Job drawing, mm, ordinate dimensions from the low corner. One solid piece. A direction names the side the tool comes from. Coordinates: 2 decimals unless noted, no trailing zeros. Order: outer loops, then holes, each group sorted by start corner. A loop starts at its lowest first (then second) coordinate and runs counter-clockwise, first axis right, second up. Notation, with made-up numbers: (40.5, -40) - (81.5, -40) arc R15 ccw to (81.5, -31) - close; hole circle Ø5 at (17, 88). An arc over 180 degrees is marked (long way). Use one line per item in the form item = value.
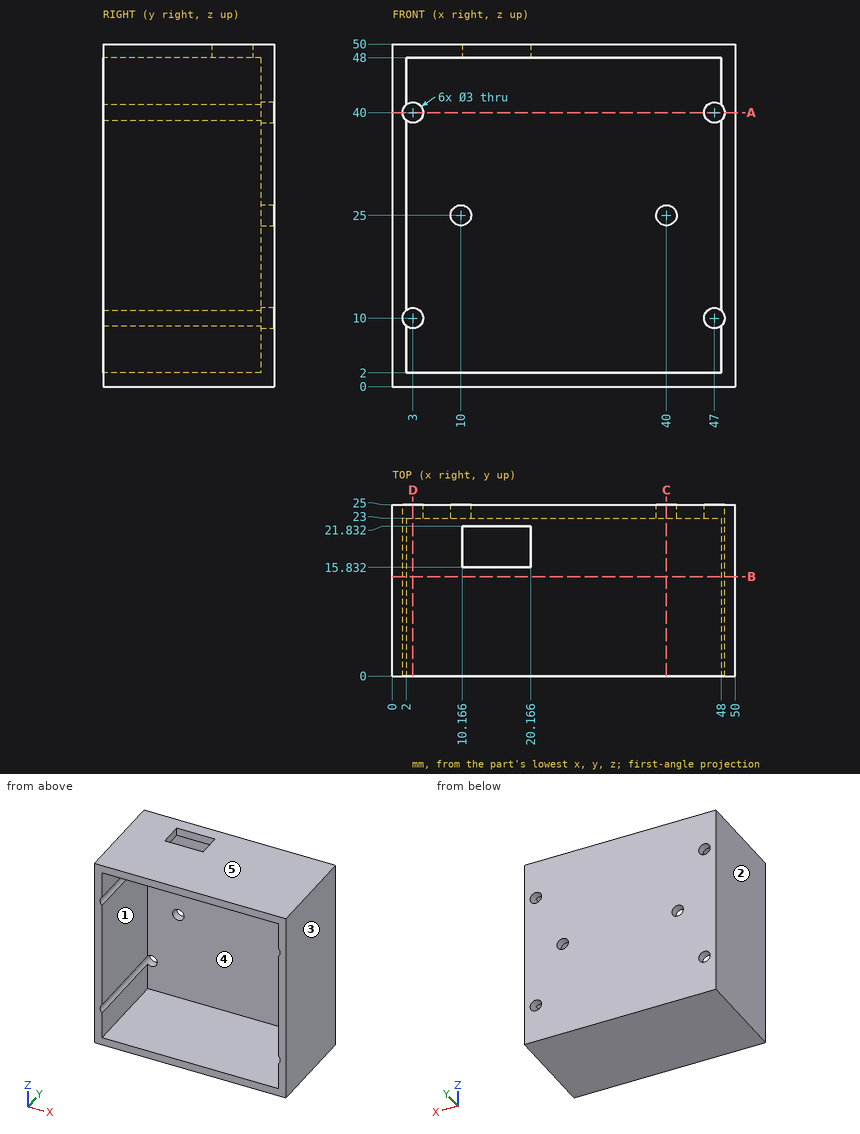
Item 1: Cut at B-B, the plane y = 14.5. Write the cut outline in (x, z), plus the area to 3 significant figures.
Derived:
outline = (0, 0) - (50, 0) - (50, 50) - (0, 50) - close; hole (2, 2) - (48, 2) - (48, 8.88) arc R1.5 ccw to (48, 11.12) - (48, 38.88) arc R1.5 ccw to (48, 41.12) - (48, 48) - (2, 48) - (2, 41.12) arc R1.5 ccw to (2, 38.88) - (2, 11.12) arc R1.5 ccw to (2, 8.88) - close
area = 381 mm²
Item 2: Two-plate mould, pull along X, no slides. Class the marked faces 3, 4 and 5: +X half, -X half, draft (parallel to the pull), parting line (faces both ways), or undercut.
Derived:
face_3 = +X half
face_4 = undercut
face_5 = draft
Item 3: 3-axis set-ups, long thin cutter, end or side, ignore diameter. For the marked faces 1 and 2: which of +Z, -Z, +X, -X, +Y, -Y reach the whole face in a straight line?
Derived:
face_1 = -Y
face_2 = +Z, -Z, -X, +Y, -Y
Item 4: Cut at C-C, the plane x = 40. Write the cut outline in (y, z), plus the area to 3 significant figures.
Derived:
outline = (0, 0) - (25, 0) - (25, 23.5) - (23, 23.5) - (23, 2) - (0, 2) - close; (0, 48) - (23, 48) - (23, 26.5) - (25, 26.5) - (25, 50) - (0, 50) - close
area = 186 mm²
Item 5: Cut at D-D, the plane x = 3. Write the cut outline in (y, z).
Derived:
outline = (0, 0) - (25, 0) - (25, 8.5) - (23, 8.5) - (23, 2) - (0, 2) - close; (0, 48) - (23, 48) - (23, 41.5) - (25, 41.5) - (25, 50) - (0, 50) - close; (23, 11.5) - (25, 11.5) - (25, 38.5) - (23, 38.5) - close
Item 6: Drop flat-ended pins along their axis: pin 1 (7.5 mm diameter, centred on y = 6.5, z = 45, fed in from -X); pin 2 (8 mm diameter, centred on x = 7, z = 22.5, fed in from -Y). Give the stop position or say it passes through.
Derived:
pin_1 = 0
pin_2 = 23
Item 7: Drill centre lines: line 1 (X direction, y = 24.2, z = 25); line 2 (Z direction, x = 3, y = 7.5). Where is each one in solid material? Low to high. Write a range as [from, to].
Derived:
line_1 = [0, 8.5], [11.5, 38.5], [41.5, 50]
line_2 = [0, 2], [48, 50]
Item 8: Cut at A-A, the plane z = 40. Write the cut outline in (x, y).
Derived:
outline = (0, 0) - (1.5, 0) - (1.5, 25) - (0, 25) - close; (4.5, 23) - (45.5, 23) - (45.5, 25) - (4.5, 25) - close; (48.5, 0) - (50, 0) - (50, 25) - (48.5, 25) - close
